```python
from build123d import *

# Parameters (mm, degrees)
SKETCH_W        = 31
SKETCH_H        = 24
PAD_DEPTH       = 22
SKETCH001_R     = 12
SKETCH001_R_2   = 1.3
POCKET_DEPTH    = 6
SKETCH002_R     = 11.25
POCKET001_DEPTH = 22.001
SKETCH003_W     = 22.5
SKETCH003_H     = 22
POCKET002_DEPTH = 11
SKETCH004_R     = 10.5
POCKET003_DEPTH = 24.001
FILLET017_R     = 0.5


with BuildPart() as part:
    # Sketch → Pad (new body)
    with BuildSketch(Plane.XY):
        Rectangle(SKETCH_W, SKETCH_H)
    extrude(amount=PAD_DEPTH)

    # Sketch001 (on Face3 of Pad) → Pocket (cut)
    with BuildSketch(Plane.XZ.offset(12)):
        with Locations((0, 15)):
            Circle(SKETCH001_R)
        with Locations((-12, 3)):
            Circle(SKETCH001_R_2)
        with Locations((12, 3)):
            Circle(SKETCH001_R_2)
        with Locations((12, 27)):
            Circle(SKETCH001_R_2)
        with Locations((-12, 27)):
            Circle(SKETCH001_R_2)
    extrude(amount=-POCKET_DEPTH, mode=Mode.SUBTRACT)

    # Sketch002 (on Face4 of Pocket) → Pocket001 (cut, through all)
    with BuildSketch(Plane(origin=(0, 0, 0), x_dir=(1, 0, 0), z_dir=(0, 0, -1))):
        Circle(SKETCH002_R)
    extrude(amount=-POCKET001_DEPTH, mode=Mode.SUBTRACT)

    # Sketch003 (on Face1 of Pocket001) → Pocket002 (cut)
    with BuildSketch(Plane(origin=(0, 12, 0), x_dir=(-1, 0, 0), z_dir=(0, 1, 0))):
        with Locations((0, 11)):
            Rectangle(SKETCH003_W, SKETCH003_H)
    extrude(amount=-POCKET002_DEPTH, mode=Mode.SUBTRACT)

    # Sketch004 (on Face6 of Pocket002) → Pocket003 (cut, through all)
    with BuildSketch(Plane.XZ.offset(12)):
        with Locations((23.47, 19.93)):
            Circle(SKETCH004_R)
    extrude(amount=-POCKET003_DEPTH, mode=Mode.SUBTRACT)

    # Fillet017
    fillet017_edges = [part.edges().sort_by_distance(p)[0] for p in [
        (-13.3, -12, 3),
        (10.7, -12, 3),
        (-15.5, 0, 0),
        (-15.5, 0, 22),
        (15.5, 0, 0),
        (11.25, 6.5, 0),
        (-11.25, 6.5, 0),
    ]]
    fillet(fillet017_edges, radius=FILLET017_R)


with BuildPart() as part_1:
    # Body placement: moved
    add(part.part.moved(Location((-9, -12, -33))))


solid = part_1.part
```
Check sheet for the modelled part. Datum: model origin and axes. Units: mm. A direction names the side the tool comes from. Round coordinates to 2 decimals unless told otherwise and drop trailing zeros. Order: outer loops, then holes, each group sorted by start corner. A loop starts at its lowest first (then second) coordinate and runs counter-clockwise, first axis right, second up.
1) Go/stop test with flat-tipped pins: pin 1 Ø2.5 at (x, z) = (3, -30) entering from -Y; pin 2 Ø3 at (x, z) = (3, -30) entering from -Y; pin 3 Ø1.5 at (y, z) = (-8, -13.5) entering from +X; pin 4 Ø12 at (x, z) = (-6, -18.5) entering from -Y. Record where each tip stops, or that it passes through.
2) Tool access check on faces 1 (the flat face through (-9, -24, -32)), 2 (the flat face through (3, -18, -30)), 3 (the flat face through (2.25, -5, -22)). Record the directions out of +Z, -Z, +X, -X, +Y, -Y that give a thin tool (end or side, any length) a straight path to the whole face; none if there is none.
3) Section check A-A (y = -8.25). Record the boundary of the cut face in (x, z).
4) Section check C-C (z = -18). Record the boundary of the cut face in (x, y).
5) Section check D-D (y = -12). Record the boundary of the cut face in (x, z).
6) Scan lines: line 1 (X direction, y = -12, z = -25.5); line 2 (Z direction, x = 5.5, y = -4.25); line 3 (X direction, y = -16, z = -16.75). Record each from-to range of solid material in increasing order.
7) Section check B-B (y = -21). Record the boundary of the cut face in (x, z).
8) Mould release check, pull along X, two halves, no side actions. Record for faces 4 (the flat face through (-24.5, -12, -22)), 5 (the flat face through (-20.25, -5, -22)), 6 (the cylindrical face through (-4.701, -22.396, -29.487)), 7 (the flat face through (6.5, -12, -26)): +X half, -X half, draft (parallel to the pull), parting line (faces both ways), or undercut.
Result:
1. pin 1: stops at y = -18
1. pin 2: stops at y = -23.9
1. pin 3: stops at x = 4.04
1. pin 4: passes through
2. face 1: +Z, -Z, +X, -X, -Y
2. face 2: -Y
2. face 3: +Z, -Z, +Y
3. outline: (-24.5, -32.5) arc R0.5 ccw to (-24, -33) - (-20.75, -33) arc R0.5 ccw to (-20.25, -32.5) - (-20.25, -11) - (-24, -11) arc R0.5 ccw to (-24.5, -11.5) - close; (2.25, -32.5) arc R0.5 ccw to (2.75, -33) - (6, -33) arc R0.5 ccw to (6.5, -32.5) - (6.5, -19.91) arc R10.5 cw to (4.18, -11) - (2.25, -11) - close
4. outline: (-24.5, -24) - (-21, -24) - (-21, -18) - (-18.52, -18) arc R11.25 cw to (-20.21, -11) - (-20.25, -11) - (-20.25, 0) - (-24.5, 0) - close; (0.52, -18) - (3, -18) - (3, -24) - (5.2, -24) - (5.2, 0) - (2.25, 0) - (2.25, -11) - (2.21, -11) arc R11.25 cw to start
5. outline: (-24.5, -32.5) arc R0.5 ccw to (-24, -33) - (-20.25, -33) - (-20.25, -11) - (-24, -11) arc R0.5 ccw to (-24.5, -11.5) - close; (2.25, -33) - (6, -33) arc R0.5 ccw to (6.5, -32.5) - (6.5, -19.91) arc R10.5 cw to (4.18, -11) - (2.25, -11) - close
6. line 1: x = -24.5 to -20.25, 2.25 to 6.5
6. line 2: z = -33 to -18.53
6. line 3: x = -24.5 to -19.51, 1.51 to 4.64
7. outline: (-24.5, -32.5) arc R0.5 ccw to (-24, -33) - (-15.75, -33) - (-15.75, -27.92) arc R12 cw to (-18.75, -11) - (-24, -11) arc R0.5 ccw to (-24.5, -11.5) - close; (-2.25, -33) - (6, -33) arc R0.5 ccw to (6.5, -32.5) - (6.5, -19.91) arc R10.5 cw to (4.18, -11) - (0.75, -11) arc R12 cw to (-2.25, -27.92) - close; hole circle Ø2.6 at (-21, -30); hole circle Ø2.6 at (3, -30)
8. face 4: -X half
8. face 5: undercut
8. face 6: undercut
8. face 7: +X half
